Work out the finished part from the listing and answer in its coordinate system (mm). A direction names the side the tool comes from. Round coordinates to 2 decimals unless told otherwise and drop trailing zeros. Order: outer loops, then holes, each group sorted by start corner. A loop starts at its lowest first (then second) coordinate and runs counter-clockwise, first axis right, second up. Notation, with made-up numbers: M 37.5,67.25 L 86.5,67.25 A37 cw 86.5,106.25 Z; hole C 65,30 d10. An arc over 180 degrees is marked long. Return JSON: item names as keys, results as strings.
from build123d import *

# Parameters (mm, degrees)
ESBO_O2_R             = 8
CORTE_EXTRUS_O1_DEPTH = 5
CORTE_EXTRUS_O2_START = -5
ESBO_O3_R             = 8
CORTE_EXTRUS_O2_DEPTH = 5
ESBO_O4_R             = 7.5
CORTE_EXTRUS_O3_DEPTH = 0.3


with BuildPart() as part:
    # Esboço1 → Revolução1 (revolve)
    with BuildSketch(Plane.XY, mode=Mode.PRIVATE) as revolu_o1_sk:
        Polygon((-5.15, 2.5), (-5.15, 9.75), (-2.65, 12.25), (-0.15, 9.75), (-0.15, 9.45), (0.15, 9.45), (0.15, 9.75), (2.65, 12.25), (5.15, 9.75), (5.15, 2.5), align=None)
    revolve(revolu_o1_sk.sketch.rotate(Axis((-5.77388535, 0, 0), (1, 0, 0)), 90), axis=Axis((-5.77388535, 0, 0), (1, 0, 0)))

    # Esboço2 → Corte-extrusão1 (cut)
    with BuildSketch(Plane(origin=(5.15, 0, 0), x_dir=(0, 0, -1), z_dir=(1, 0, 0))):
        Circle(ESBO_O2_R)
    extrude(amount=-CORTE_EXTRUS_O1_DEPTH, mode=Mode.SUBTRACT)

    # Esboço3 → Corte-extrusão2 (cut)
    with BuildSketch(Plane.ZY.offset(5.15).offset(CORTE_EXTRUS_O2_START)):
        with Locations(Location((0, 0, 0), (0, 0, 180))):
            Circle(ESBO_O3_R)
    extrude(amount=CORTE_EXTRUS_O2_DEPTH, mode=Mode.SUBTRACT)

    # Esboço4 → Corte-extrusão3 (cut)
    with BuildSketch(Plane.ZY.offset(0.15)):
        Circle(ESBO_O4_R)
    extrude(amount=-CORTE_EXTRUS_O3_DEPTH, mode=Mode.SUBTRACT)


solid = part.part
Item 1: The mould has two halves that part along X. Classify faces 5 (the conical face through (-0.271, -2.965, 9.416)), 6 (the flat face through (0.15, -6, -5)), 7 (the cylindrical face through (0, -7.32, -1.63)), 8 (the cylindrical face through (0, -7.97, 5.08)): pulls with the +X half, pulls with the -X half, needs draft (parallel to the pull), parting line crosses it, or undercut.
Output:
{"face 5": "undercut", "face 6": "pulls with the +X half", "face 7": "needs draft", "face 8": "undercut"}
Item 2: Find section C-C (x = 2). Determine the outline of the cut face in (y, z), plus the area to 3 significant figures.
Output:
{"outline": "C 0,0 d23.2; hole C 0,0 d16", "area": "222 mm^2"}
Item 3: Find section A-A (y = 0). Determine the outline of the cut face in (x, z), plus the area to 3 significant figures.
Output:
{"outline": "M -5.15,-9.75 L -2.65,-12.25 L -0.15,-9.75 L -0.15,-9.45 L 0.15,-9.45 L 0.15,-9.75 L 2.65,-12.25 L 5.15,-9.75 L 5.15,-8 L 0.15,-8 L 0.15,-7.5 L -0.15,-7.5 L -0.15,-8 L -5.15,-8 Z; M -5.15,8 L -0.15,8 L -0.15,7.5 L 0.15,7.5 L 0.15,8 L 5.15,8 L 5.15,9.75 L 2.65,12.25 L 0.15,9.75 L 0.15,9.45 L -0.15,9.45 L -0.15,9.75 L -2.65,12.25 L -5.15,9.75 Z", "area": "61.2 mm^2"}
Item 4: Each of these flat-tipped pins is pushed along its axis until it touches: pin 1 (1 mm diameter, centred on x = 1, y = 1, fed in from +Z); pin 2 (3 mm diameter, centred on x = 1, y = 3.5, fed in from +Z); pin 3 (1.5 mm diameter, centred on x = 0.5, z = 0, fed in from -Y). Where does it stop, or does it pass through?
Output:
{"pin 1": "stops at z = 11.06", "pin 2": "stops at z = 11.64", "pin 3": "stops at y = -10.85"}
Item 5: Which of the six approach directions +Z, -Z, +X, -X, +Y, -Y give full straight-line access (tool end or side, diameter ignored) to faces 1 (the flat face through (-0.15, 6, -5)), 2 (the flat face through (5.15, -3.7, -7.3)), 3 (the conical face through (0.31, -2.98, 9.45)), 4 (the cylindrical face through (2.69, -7.81, 1.73))?
Output:
{"face 1": "-X", "face 2": "+Z, -Z, +X, +Y, -Y", "face 3": "none", "face 4": "+X"}
Item 6: Find section D-D (x = -0.5). Determine the outline of the cut face in (y, z), plus the area to 3 significant figures.
Output:
{"outline": "C 0,0 d20.2; hole C 0,0 d16", "area": "119 mm^2"}
Item 7: Consider line 1 along Y through (x, z) = (0.05, 0); line 2 along X through (y, z) = (4.5, -8.5); line 3 along Y through (x, z) = (-3.95, 0). Determine where each line is inside the solid, lowest interval first. Write a range as [from, to].
Output:
{"line 1": "y = [-9.45, -7.5], [7.5, 9.45]", "line 2": "x = [-5.15, -0.15], [0.15, 5.15]", "line 3": "y = [-10.95, -8], [8, 10.95]"}
